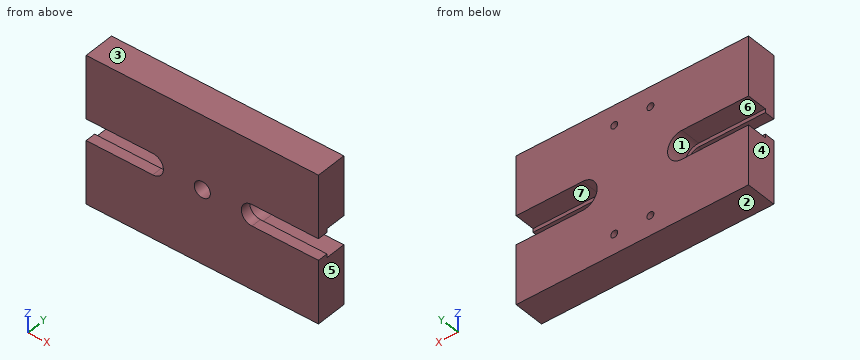
Autodesk Inventor part; units mm, degrees
ref_plane "YZ Plane" through (0, 0, 0) normal (1, 0, 0) x (0, 1, 0)
ref_plane "XZ Plane" through (0, 0, 0) normal (0, 1, 0) x (-1, 0, 0)
ref_plane "XY Plane" through (0, 0, 0) normal (0, 0, 1) x (1, 0, 0)
sketch "Sketch1" plane through (0, 0, 0) normal (0, 1, 0) x (-1, 0, 0)
  line L0 (22.9489, 20.701) -> (-22.9489, 20.701)
  line L1 (-22.9489, 20.701) -> (-22.9489, -20.701)
  line L2 (-22.9489, -20.701) -> (22.9489, -20.701)
  line L3 (22.9489, -20.701) -> (22.9489, 20.701)
  line L4 (22.9489, 20.701) -> (-22.9489, -20.701) construction
  line L5 (-22.9489, 20.701) -> (22.9489, -20.701) construction
  point P0 (0, 0)
  dimension "d0" = 45.8978
  dimension "d1" = 41.402
extrude "Extrusion1" add sketch "Sketch1" along normal blind 9.525
hole "Hole1" at (0, 0, 0) direction (0, 1, 0) diameter 4.9784 depth 6.35
sketch "Sketch11" plane through (-22.9489, 0, 20.701) normal (0, 0, 1) x (1, 0, 0)
  line L0 (45.8978, 9.525) -> (0, 9.525)
  line L1 (45.8978, 0) -> (0, 0)
  line L2 (0, 9.525) -> (45.8978, 9.525)
  line L3 (45.8978, 9.525) -> (45.8978, 0)
  line L4 (45.8978, 0) -> (0, 0)
  line L5 (0, 0) -> (0, 9.525)
  point P0 (22.9489, 0)
extrude "Extrusion6" cut sketch "Sketch11" against normal blind 3.175
sketch "Sketch12" plane through (22.9489, 0, -20.701) normal (0, 0, -1) x (-1, 0, 0)
  line L0 (0, 9.525) -> (45.8978, 9.525)
  line L1 (45.8978, 0) -> (45.8978, 9.525)
  line L2 (0, 9.525) -> (45.8978, 9.525)
  line L3 (45.8978, 9.525) -> (45.8978, 0)
  line L4 (45.8978, 0) -> (0, 0)
  line L5 (0, 0) -> (0, 9.525)
  point P0 (22.9489, 0)
extrude "Extrusion7" cut sketch "Sketch12" against normal blind 3.175
sketch "Sketch13" plane through (22.9489, 0, 17.526) normal (1, 0, 0) x (0, 0, -1)
  line L0 (0, 9.525) -> (0, 0)
  line L1 (35.052, 0) -> (0, 0)
  line L2 (0, 9.525) -> (35.052, 9.525)
  line L3 (35.052, 9.525) -> (35.052, 0)
  line L4 (35.052, 0) -> (0, 0)
  line L5 (0, 0) -> (0, 9.525)
  point P0 (17.526, 0)
extrude "Extrusion8" add sketch "Sketch13" along normal blind 12.9426
sketch "Sketch14" plane through (-22.9489, 0, 17.526) normal (-1, 0, 0) x (0, 0, 1)
  line L0 (-35.052, 9.525) -> (0, 9.525)
  line L1 (-35.052, 9.525) -> (0, 9.525)
  line L2 (0, 9.525) -> (0, 0)
  line L3 (0, 0) -> (-35.052, 0)
  line L4 (-35.052, 0) -> (-35.052, 9.525)
  point P0 (-17.526, 0)
extrude "Extrusion9" add sketch "Sketch14" along normal blind 12.9426
sketch "Sketch2" plane through (0, 9.525, 0) normal (0, 1, 0) x (1, 0, 0)
  line L0 (22.9489, -20.701) -> (22.9489, 20.701)
  line L1 (-22.9489, -20.701) -> (22.9489, -20.701)
  line L2 (22.9489, 20.701) -> (-22.9489, 20.701)
  line L3 (-22.9489, 20.701) -> (-22.9489, -20.701)
  arc A0 (-15.3289, -3.302) -> (-15.3289, 3.302) centre (-15.3289, 0) ccw
  line L4 (-15.3289, -3.302) -> (-22.9489, -3.302)
  line L5 (-15.3289, 3.302) -> (-22.9489, 3.302)
  arc A1 (15.3289, 3.302) -> (15.3289, -3.302) centre (15.3289, 0) ccw
  line L6 (15.3289, 3.302) -> (22.9489, 3.302)
  line L7 (15.3289, -3.302) -> (22.9489, -3.302)
  line L8 (-22.9489, 4.445) -> (-15.3289, 4.445)
  arc A2 (-15.3289, -4.445) -> (-15.3289, 4.445) centre (-15.3289, 0) ccw
  line L9 (-15.3289, -4.445) -> (-22.9489, -4.445)
  line L10 (22.9489, 4.445) -> (15.3289, 4.445)
  arc A3 (15.3289, 4.445) -> (15.3289, -4.445) centre (15.3289, 0) ccw
  line L11 (15.3289, -4.445) -> (22.9489, -4.445)
  line L12 (22.9489, -4.445) -> (35.8915, -4.445)
  line L13 (35.8915, -17.526) -> (35.8915, 17.526)
  line L14 (22.9489, -3.302) -> (35.8915, -3.302)
  line L15 (22.9489, 3.302) -> (35.8915, 3.302)
  line L16 (22.9489, 4.445) -> (35.8915, 4.445)
  line L17 (-22.9489, 4.445) -> (-35.8915, 4.445)
  line L18 (-35.8915, -17.526) -> (-35.8915, 17.526)
  line L19 (-22.9489, 3.302) -> (-25.4, 3.302)
  line L20 (-22.9489, -3.302) -> (-35.8915, -3.302)
  line L21 (-22.9489, -4.445) -> (-35.8915, -4.445)
  line L22 (-25.4, 3.302) -> (-35.8915, 3.302)
  point P0 (22.9489, 0)
  point P1 (-22.9489, 0)
  dimension "d21" = 1.143
extrude "Extrusion10" cut sketch "Sketch2" against normal through all contours L7 A1 L6 L0 | L0 L15 L13 L14 | L20 L18 L22 L19 L3 | L3 L5 A0 L4
extrude "Extrusion11" cut sketch "Sketch2" against normal blind 6.35 contours L11 A3 L10 L0 L6 A1 L7 | L0 L14 L13 L12 | L21 L18 L20 L3 | L3 L4 A0 L5 L8 A2 L9 | L0 L16 L13 L15 | L19 L22 L18 L17 L3
sketch "Sketch15" plane through (22.9489, 0, -17.526) normal (0, 0, -1) x (-1, 0, 0)
  line L0 (-12.9426, 9.525) -> (-12.9426, 0)
  line L1 (58.8404, 9.525) -> (58.8404, 0)
  line L2 (-12.9426, 9.525) -> (58.8404, 9.525)
  line L3 (58.8404, 9.525) -> (58.8404, 0)
  line L4 (58.8404, 0) -> (-12.9426, 0)
  line L5 (-12.9426, 0) -> (-12.9426, 9.525)
  point P0 (22.9489, 0)
extrude "Extrusion12" add sketch "Sketch15" along normal blind 5.285
sketch "Sketch16" plane through (-22.9489, 0, 17.526) normal (0, 0, 1) x (1, 0, 0)
  line L0 (-12.9426, 3.175) -> (-12.9426, 9.525)
  line L1 (58.8404, 0) -> (-12.9426, 0)
  line L2 (-12.9426, 9.525) -> (58.8404, 9.525)
  line L3 (58.8404, 9.525) -> (58.8404, 0)
  line L4 (58.8404, 0) -> (-12.9426, 0)
  line L5 (-12.9426, 0) -> (-12.9426, 9.525)
  point P0 (22.9489, 0)
extrude "Extrusion13" add sketch "Sketch16" along normal blind 5.285
sketch "Sketch19" plane through (0, 9.525, 0) normal (0, 1, 0) x (1, 0, 0)
  line L0 (-35.8915, 3.302) -> (-35.8915, 22.811)
  line L1 (-35.8915, 22.811) -> (-5.5893, 22.811)
  line L2 (-35.8915, 16.6642) -> (-35.8915, 22.811)
  line L3 (35.8915, 22.811) -> (-35.8915, 22.811)
  line L4 (35.8915, 22.811) -> (5.5893, 22.811)
  line L5 (35.8915, 16.6642) -> (35.8915, 22.811)
  line L6 (35.8915, -22.811) -> (-35.8915, -22.811)
  line L7 (-35.8915, -22.811) -> (-5.5893, -22.811)
  line L8 (-35.8915, -16.6642) -> (-35.8915, -22.811)
  line L9 (35.8915, -22.811) -> (5.5893, -22.811)
  line L10 (35.8915, -16.6642) -> (35.8915, -22.811)
  point P0 (0, 0)
  point P1 (-5.5893, 16.6642)
  point P2 (5.5893, 16.6642)
  point P3 (-5.5893, -16.6642)
  point P4 (5.5893, -16.6642)
hole "Hole2" at (-5.5893, 9.525, 16.6642) at (5.5893, 9.525, 16.6642) at (-5.5893, 9.525, -16.6642) at (5.5893, 9.525, -16.6642) direction (0, -1, 0) diameter 2.1565 depth 6.35
properties part number "bottomblock_al_ledgereod" material "Aluminum 6061"
Work out the finished part from the listing and answer in its coordinate system (mm). Face numbers are marked on the shaded views. A direction names the side the tool comes from. Round coordinates to 2 decimals unless told otherwise and drop trailing zeros. Write each loop counter-clockwise with the first axis right and the second up, starting at its lowest first coordinate (ties: lowest second). Pieces come first, ordered by that corner, then holes. Notation, with made-up numbers: (-16.75, -14) - (-8.75, -14) arc R21 ccw to (-8.75, 24) - close; hole circle Ø9 at (-27, 34.25). An arc over 180 degrees is marked (long way). Answer in a Markdown table with one row per item. Add a question column.
1. Find the intervals of material crossed by line 1 along Z through (x, y) = (0, 5); line 2 along Z through (x, y) = (5.5, 4.75); line 3 along Z through (x, y) = (-29, 1.5), in increasing order. Write a range as from..to.
2. For the marked faces 5, 6 and 7, determine the directions among +Z, -Z, +X, -X, +Y, -Y from which every point of the face is accessible in a straight line to the end or side of a thin tool.
3. A cutting plane is placed at B-B, the plane y = 2. Determine the outline of the cut face in (x, z).
4. A cutting plane is placed at A-A, the plane x = 21. Determine the outline of the cut face in (y, z) (3 decimals).
5. A cutting plane is placed at D-D, the plane y = 8. Determine the outline of the cut face in (x, z) (1 decimal), and give its area (3 significant figures).
6. Given pin 1 (1.7 mm diameter, centred on x = -6, z = 17, fed in from +Y) (3 decimals); pin 2 (1.1 mm diameter, centred on x = 5.5, z = 16.5, fed in from +Y) (3 decimals), each flat-ended and moving along its own axis, determine where each tip first touches the part or whether it passes through.
7. The mould has two halves that part along Z. Classify the marked faces 1, 2, 3 and 4: +Z half, -Z half, draft (parallel to the pull), parting line (faces both ways), or undercut.
8. A cutting plane is placed at C-C, the plane z = 0. Determine the outline of the cut face in (x, y) (3 decimals), and give its area (3 significant figures).
Worked out:
| question | item | result |
|---|---|---|
| 1 | line 1 | -22.81..-2.49, 2.49..22.81 |
| 1 | line 2 | -22.81..-17.74, -15.59..15.59, 17.74..22.81 |
| 1 | line 3 | -22.81..-3.3, 3.3..22.81 |
| 2 | face 5 | +Z, -Z, +X, +Y, -Y |
| 2 | face 6 | -X, +Y |
| 2 | face 7 | +X, +Y |
| 3 | outline | (-35.89, -22.81) - (35.89, -22.81) - (35.89, -3.3) - (15.33, -3.3) arc R3.3 cw to (15.33, 3.3) - (35.89, 3.3) - (35.89, 22.81) - (-35.89, 22.81) - (-35.89, 3.3) - (-15.33, 3.3) arc R3.3 cw to (-15.33, -3.3) - (-35.89, -3.3) - close; hole circle Ø4.98 at (0, 0) |
| 4 | outline | (0, -22.811) - (9.525, -22.811) - (9.525, -4.445) - (3.175, -4.445) - (3.175, -3.302) - (0, -3.302) - close; (0, 3.302) - (3.175, 3.302) - (3.175, 4.445) - (9.525, 4.445) - (9.525, 22.811) - (0, 22.811) - close |
| 5 | outline | (-35.9, -22.8) - (35.9, -22.8) - (35.9, -4.4) - (15.3, -4.4) arc R4.4 cw to (15.3, 4.4) - (35.9, 4.4) - (35.9, 22.8) - (-35.9, 22.8) - (-35.9, 4.4) - (-15.3, 4.4) arc R4.4 cw to (-15.3, -4.4) - (-35.9, -4.4) - close; hole circle Ø2.2 at (-5.6, -16.7); hole circle Ø2.2 at (-5.6, 16.7); hole circle Ø2.2 at (5.6, -16.7); hole circle Ø2.2 at (5.6, 16.7) |
| 5 | area | 2,830 mm^2 |
| 6 | pin 1 | y = 9.525 |
| 6 | pin 2 | y = 3.175 |
| 7 | face 1 | undercut |
| 7 | face 2 | -Z half |
| 7 | face 3 | +Z half |
| 7 | face 4 | draft |
| 8 | outline | (-12.027, 0) - (-2.489, 0) - (-2.489, 6.35) - (2.489, 6.35) - (2.489, 0) - (12.027, 0) - (12.027, 3.175) - (10.884, 3.175) - (10.884, 9.525) - (-10.884, 9.525) - (-10.884, 3.175) - (-12.027, 3.175) - close |
| 8 | area | 183 mm^2 |
